from build123d import *

# Parameters (mm, degrees)
BOSS_EXTRUDE1_DEPTH = 39.9
SKETCH2_R           = 1.5
CUT_EXTRUDE1_DEPTH  = 4
CUT_EXTRUDE2_DEPTH  = 5.2
CUT_EXTRUDE3_START  = -39.9
CUT_EXTRUDE3_DEPTH  = 5.2
BOSS_EXTRUDE2_DEPTH = 1
BOSS_EXTRUDE3_START = -39.9
BOSS_EXTRUDE3_DEPTH = 1
SKETCH5_W           = 9.2
SKETCH5_H           = 29.5
CUT_EXTRUDE4_DEPTH  = 0.11


with BuildPart() as part:
    # Sketch1 → Boss-Extrude1 (new body)
    with BuildSketch(Plane.XY):
        Polygon((4.5, 4.5), (-4.5, 4.5), (-4.5, 0), (-10, 0), (-10, 8), (10, 8), (10, 0), (4.5, 0), align=None)
    extrude(amount=BOSS_EXTRUDE1_DEPTH)

    # Sketch2 → Cut-Extrude1 (cut)
    with BuildSketch(Plane(origin=(0, 8, 0), x_dir=(1, 0, 0), z_dir=(0, 1, 0))):
        with Locations(Location((-7.5, -11.95, 0), (0, 0, 180))):
            Circle(SKETCH2_R)
        with Locations((7.5, -11.95)):
            Circle(SKETCH2_R)
        with Locations(Location((7.5, -27.95, 0), (0, 0, 180))):
            Circle(SKETCH2_R)
        with Locations((-7.5, -27.95)):
            Circle(SKETCH2_R)
    extrude(amount=-CUT_EXTRUDE1_DEPTH, mode=Mode.SUBTRACT)

    # Sketch3 → Cut-Extrude2 (cut)
    with BuildSketch(Plane(origin=(0, 0, 0), x_dir=(-1, 0, 0), z_dir=(0, 0, -1))):
        Polygon((4.5, 0), (10, 0), (10, 8), (-10, 8), (-10, 0), (-4.5, 0), (-4.5, 4.5), (4.5, 4.5), align=None)
        Polygon((4.6, 0.1), (9.9, 0.1), (9.9, 7.9), (-9.9, 7.9), (-9.9, 0.1), (-4.6, 0.1), (-4.6, 4.6), (4.6, 4.6), align=None, mode=Mode.SUBTRACT)
    extrude(amount=-CUT_EXTRUDE2_DEPTH, mode=Mode.SUBTRACT)

    # Sketch3<3> → Cut-Extrude3 (cut)
    with BuildSketch(Plane(origin=(0, 0, 0), x_dir=(-1, 0, 0), z_dir=(0, 0, -1)).offset(CUT_EXTRUDE3_START)):
        Polygon((10, 0), (10, 8), (-10, 8), (-10, 0), (-4.5, 0), (-4.5, 4.5), (4.5, 4.5), (4.5, 0), align=None)
        Polygon((9.9, 0.1), (9.9, 7.9), (-9.9, 7.9), (-9.9, 0.1), (-4.6, 0.1), (-4.6, 4.6), (4.6, 4.6), (4.6, 0.1), align=None, mode=Mode.SUBTRACT)
    extrude(amount=CUT_EXTRUDE3_DEPTH, mode=Mode.SUBTRACT)

    # Sketch4 → Boss-Extrude2 (add)
    with BuildSketch(Plane(origin=(0, 0, 0), x_dir=(-1, 0, 0), z_dir=(0, 0, -1))):
        Polygon((4.5, 4.5), (4.5, 0), (10, 0), (10, 8), (-10, 8), (-10, 0), (-4.5, 0), (-4.5, 4.5), align=None)
    extrude(amount=-BOSS_EXTRUDE2_DEPTH)

    # Sketch4<2> → Boss-Extrude3 (add)
    with BuildSketch(Plane(origin=(0, 0, 0), x_dir=(-1, 0, 0), z_dir=(0, 0, -1)).offset(BOSS_EXTRUDE3_START)):
        Polygon((4.5, 4.5), (4.5, 0), (10, 0), (10, 8), (-10, 8), (-10, 0), (-4.5, 0), (-4.5, 4.5), align=None)
    extrude(amount=BOSS_EXTRUDE3_DEPTH)

    # Sketch5 → Cut-Extrude4 (cut)
    with BuildSketch(Plane(origin=(0, 8, 0), x_dir=(1, 0, 0), z_dir=(0, 1, 0))):
        with Locations((0, -19.95)):
            Rectangle(SKETCH5_W, SKETCH5_H)
    extrude(amount=-CUT_EXTRUDE4_DEPTH, mode=Mode.SUBTRACT)


solid = part.part
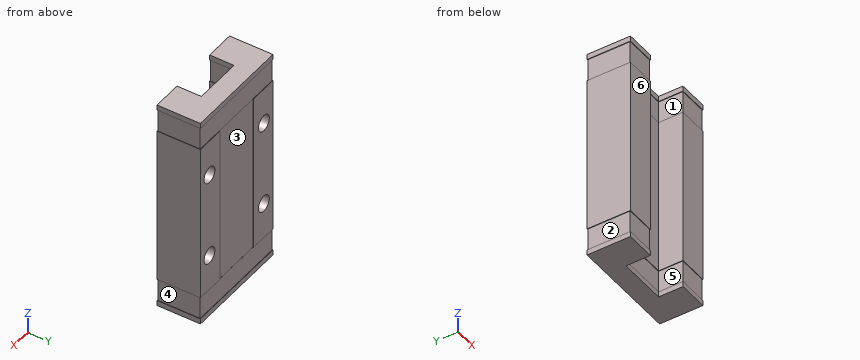
Source: CAD feature listing. Evaluate the final solid. Frame: model axes, mm. Face numbers are marked on the shaded views. A direction names the side the tool comes from. Coordinates: 2 decimals unless noted, no trailing zeros. Order: outer loops, then holes, each group sorted by start corner. A loop starts at its lowest first (then second) coordinate and runs counter-clockwise, first axis right, second up.
Item 1: Cut plane A-A (z = 7). Return loops of the section in (x, y).
Output values:
outline: (-10, 0) - (-4.5, 0) - (-4.5, 4.5) - (4.5, 4.5) - (4.5, 0) - (10, 0) - (10, 8) - (4.6, 8) - (4.6, 7.89) - (-4.6, 7.89) - (-4.6, 8) - (-10, 8) - close
Item 2: Set-up query: the marked faces 1, 2 and 3. Return all of +Z, -Z, +X, -X, +Y, -Y with unobstructed straight access to the full face (end or side cutting, diameter ignored); none if empty.
Output values:
face 1: -Y
face 2: -X, +Y, -Y
face 3: +Y
Item 3: Cut plane B-B (y = 6.5). Return loops of the section in (x, z), plus the area to 3 significant figures.
Output values:
outline: (-10, 0) - (10, 0) - (10, 1) - (9.9, 1) - (9.9, 5.2) - (10, 5.2) - (10, 34.7) - (9.9, 34.7) - (9.9, 38.9) - (10, 38.9) - (10, 39.9) - (-10, 39.9) - (-10, 38.9) - (-9.9, 38.9) - (-9.9, 34.7) - (-10, 34.7) - (-10, 5.2) - (-9.9, 5.2) - (-9.9, 1) - (-10, 1) - close; hole circle Ø3 at (-7.5, 11.95); hole circle Ø3 at (-7.5, 27.95); hole circle Ø3 at (7.5, 11.95); hole circle Ø3 at (7.5, 27.95)
area: 768 mm2
Item 4: Pull-direction query (X, two-part tool) for the marked faces 4, 5 and 6; classes: pulls with the +X half, pulls with the -X half, needs draft (parallel to the pull), parting line crosses it, or undercut.
Output values:
face 4: pulls with the +X half
face 5: undercut
face 6: needs draft
Item 5: Cut plane D-D (z = 11.95). Return loops of the section in (x, y), plus the area to 3 significant figures.
Output values:
outline: (-10, 0) - (-4.5, 0) - (-4.5, 4.5) - (4.5, 4.5) - (4.5, 0) - (10, 0) - (10, 8) - (9, 8) - (9, 4) - (6, 4) - (6, 8) - (4.6, 8) - (4.6, 7.89) - (-4.6, 7.89) - (-4.6, 8) - (-6, 8) - (-6, 4) - (-9, 4) - (-9, 8) - (-10, 8) - close
area: 94.5 mm2
Item 6: First-contact query: P1, Ø1.3, axis at y = 5.5, z = 4, coming from the +X side; P2, Ø1.3, axis at x = -7, z = 4, coming from the -Y side; P3, Ø1.5, axis at x = -7, z = 27.5, coming from the +Y side. Flat tips, straight axial feed; report the tip coordinate or a pass-through.
Output values:
P1: stops at x = 9.9
P2: stops at y = 0.1
P3: stops at y = 4
Item 7: Material intervals for line 1 (Z direction, x = -7.5, y = 5.5); line 2 (X direction, y = 2.75, z = 25.5); line 3 (X direction, y = 2, z = 4), sorted ascending.
Output values:
line 1: z = 0 to 10.45, 13.45 to 26.45, 29.45 to 39.9
line 2: x = -10 to -4.5, 4.5 to 10
line 3: x = -9.9 to -4.6, 4.6 to 9.9
